```python
from build123d import *

# Parameters (mm, degrees)
SKETCH1_R           = 75
BOSS_EXTRUDE1_DEPTH = 5
SKETCH2_R           = 3
CUT_EXTRUDE1_DEPTH  = 5
CIRPATTERN1_COUNT   = 4
SKETCH4_R           = 55
SKETCH4_R_2         = 53
CUT_EXTRUDE3_DEPTH  = 1.3208
SKETCH5_R           = 75
SKETCH5_R_2         = 60
CUT_EXTRUDE4_DEPTH  = 5


with BuildPart() as part:
    # Sketch1 → Boss-Extrude1 (new body)
    with BuildSketch(Plane.XY):
        Circle(SKETCH1_R)
    extrude(amount=BOSS_EXTRUDE1_DEPTH)

    # Sketch2 → Cut-Extrude1 (cut)
    with BuildSketch(Plane.XY.offset(5)):
        with Locations((28.284271247, 28.284271247)):
            Circle(SKETCH2_R)
    cut_extrude1 = extrude(amount=-CUT_EXTRUDE1_DEPTH, mode=Mode.SUBTRACT)

    # CirPattern1: Cut-Extrude1 ×4 about axis
    cirpattern1_axis = Axis((0, 0, 0), (0, 0, 1))
    for i in range(1, CIRPATTERN1_COUNT):
        add(cut_extrude1.rotate(cirpattern1_axis, i * 360 / CIRPATTERN1_COUNT), mode=Mode.SUBTRACT)

    # Sketch4 → Cut-Extrude3 (cut)
    with BuildSketch(Plane.XY.offset(5)):
        Circle(SKETCH4_R)
        Circle(SKETCH4_R_2, mode=Mode.SUBTRACT)
    extrude(amount=-CUT_EXTRUDE3_DEPTH, mode=Mode.SUBTRACT)

    # Sketch5 → Cut-Extrude4 (cut)
    with BuildSketch(Plane.XY.offset(5)):
        Circle(SKETCH5_R)
        Circle(SKETCH5_R_2, mode=Mode.SUBTRACT)
    extrude(amount=-CUT_EXTRUDE4_DEPTH, mode=Mode.SUBTRACT)


solid = part.part
```
Can you work these out from the model? Positions are in its coordinate system, mm. A direction names the side the tool comes from. Coordinates: 2 decimals unless noted, no trailing zeros. Order: outer loops, then holes, each group sorted by start corner. A loop starts at its lowest first (then second) coordinate and runs counter-clockwise, first axis right, second up. Notation, with made-up numbers: (-30.75, 78.5) -> (4.25, 78.5) arc R3 ccw to (4.25, 83.5) -> close; hole circle Ø11 at (39, -7). An arc over 180 degrees is marked (long way). Write each question's results on one line, items separated by ' | '.
Item 1: I'm going to push flat-ended pins straight in: pin 1 Ø3.5 at (x, y) = (28.28, 28.28) entering from -Z; pin 2 Ø1 at (y, z) = (43, 1) entering from +X. Where does each tip first touch, or does it pass through?
Results are:
pin 1: through | pin 2: x = 42.35
Item 2: I want a section at B-B, the plane z = 2.35. Write out the boundary of the cut face in (x, y), then the cut area to 3 significant figures.
Results are:
outline: circle Ø120 at (0, 0); hole circle Ø6 at (-28.28, -28.28); hole circle Ø6 at (-28.28, 28.28); hole circle Ø6 at (28.28, -28.28); hole circle Ø6 at (28.28, 28.28) | area: 11,200 mm²
Item 3: If we mould it in two halves opening along Y, with no side actions, what happens to faces 1 (the face through (26, -49, 5)), 2 (the face through (-45, 29, 3.679)), 3 (the face through (-59.94, 2.64, 2.54))? For each: +Y half, -Y half, draft (parallel to the pull), parting line (faces both ways), or undercut.
Results are:
face 1: draft | face 2: undercut | face 3: parting line
Item 4: Which directions (+Z, -Z, +X, -X, +Y, -Y) give clear straight access to the entire face, cutting with the end or side of a thin tool? Please do faces 4 (the face through (31.056, 27.135, 2.535)), 5 (the face through (-11.923, -53.692, 4.349)).
Results are:
face 4: +Z, -Z | face 5: +Z
Item 5: I want a section at A-A, the plane y = -47.5. Write out the boundary of the cut face in (x, z).
Results are:
outline: (-36.66, 0) -> (36.66, 0) -> (36.66, 5) -> (27.73, 5) -> (27.73, 3.68) -> (23.51, 3.68) -> (23.51, 5) -> (-23.51, 5) -> (-23.51, 3.68) -> (-27.73, 3.68) -> (-27.73, 5) -> (-36.66, 5) -> close
Item 6: If I drill on line 1 along Y through (x, z) = (0, 4.1); line 2 along X through (y, z) = (30, 2.4); line 3 along Y through (x, z) = (45.5, 4.7), over which ranges is the centre line in solid material (lowest first)?
Results are:
line 1: -60 to -55, -53 to 53, 55 to 60 | line 2: -51.96 to -30.75, -25.82 to 25.82, 30.75 to 51.96 | line 3: -39.11 to -30.9, -27.18 to 27.18, 30.9 to 39.11
Item 7: I want a section at C-C, the plane x = -19.5. Write out the boundary of the cut face in (y, z).
Results are:
outline: (-56.74, 0) -> (56.74, 0) -> (56.74, 5) -> (51.43, 5) -> (51.43, 3.68) -> (49.28, 3.68) -> (49.28, 5) -> (-49.28, 5) -> (-49.28, 3.68) -> (-51.43, 3.68) -> (-51.43, 5) -> (-56.74, 5) -> close
